Verification items for the finished model (mm, model axes). A direction names the side the tool comes from. Round coordinates to 2 decimals unless told otherwise and drop trailing zeros. Loops run counter-clockwise (first coordinate to the right, second up) from the corner with the lowest first, then second, coordinate; pieces in that order, holes last. Notation, with made-up numbers: (89.25, -36.5) -> (98.25, -36.5) arc R6 cw to (98.25, -25.5) -> close; hole circle Ø5 at (-11, 42). An arc over 180 degrees is marked (long way). Write item = value, one per line.
```python
from build123d import *

# Parameters (mm, degrees)
SKETCH1_R           = 78.35
SKETCH1_R_2         = 4
SKETCH1_R_3         = 3
BOSS_EXTRUDE1_DEPTH = 5
SKETCH2_R           = 78.35
SKETCH2_R_2         = 75.35
BOSS_EXTRUDE2_DEPTH = 8
SKETCH3_W           = 100
SKETCH3_H           = 100
CUT_EXTRUDE1_DEPTH  = 3


with BuildPart() as part:
    # Sketch1 → Boss-Extrude1 (new body)
    with BuildSketch(Plane(origin=(0, 0, 0), x_dir=(1, 0, 0), z_dir=(0, 1, 0))):
        with Locations(Location((0, 0, 0), (0, 0, 270))):
            Circle(SKETCH1_R)
        with Locations(Location((-62.5, 0, 0), (0, 0, 270))):
            Circle(SKETCH1_R_2, mode=Mode.SUBTRACT)
        with Locations(Location((62.5, 0, 0), (0, 0, 270))):
            Circle(SKETCH1_R_2, mode=Mode.SUBTRACT)
        with Locations(Location((0, 62.5, 0), (0, 0, 270))):
            Circle(SKETCH1_R_3, mode=Mode.SUBTRACT)
        with Locations(Location((0, -62.5, 0), (0, 0, 270))):
            Circle(SKETCH1_R_3, mode=Mode.SUBTRACT)
    extrude(amount=BOSS_EXTRUDE1_DEPTH)

    # Sketch2 → Boss-Extrude2 (add)
    with BuildSketch(Plane(origin=(0, 5, 0), x_dir=(1, 0, 0), z_dir=(0, 1, 0))):
        with Locations(Location((0, 0, 0), (0, 0, 270))):
            Circle(SKETCH2_R)
        with Locations(Location((0, 0, 0), (0, 0, 270))):
            Circle(SKETCH2_R_2, mode=Mode.SUBTRACT)
    extrude(amount=BOSS_EXTRUDE2_DEPTH)

    # Sketch3 → Cut-Extrude1 (cut)
    with BuildSketch(Plane(origin=(0, 5, 0), x_dir=(1, 0, 0), z_dir=(0, 1, 0))):
        Rectangle(SKETCH3_W, SKETCH3_H)
    extrude(amount=-CUT_EXTRUDE1_DEPTH, mode=Mode.SUBTRACT)


solid = part.part
```
(1) Draft check along X on faces 1 (the face through (64, 13, -41)), 2 (the face through (-1.8, 2.5, -64.9)), 3 (the face through (23.534, 6.409, 74.732)). Enter one of: released by +X, released by -X, zero draft, split by the parting line, or undercut.
Filled sheet:
face_1 = zero draft
face_2 = undercut
face_3 = split by the parting line
(2) Set-up check for faces 4 (the face through (74.71, 8.94, -9.81)), 5 (the face through (1, 0, -1)): record each of +Z, -Z, +X, -X, +Y, -Y from which the full face is reachable in a straight line by a thin tool's end or side.
Filled sheet:
face_4 = +Y
face_5 = +Z, -Z, +X, -X, -Y
(3) Material ranges on probe 1 along X at (y, z) = (1.25, 0); probe 2 along X at (y, z) = (3.2, 0); probe 3 along X at (y, z) = (9.5, 0), recorded low to high. Write a range as from..to.
Filled sheet:
probe_1 = -78.35..-66.5, -58.5..58.5, 66.5..78.35
probe_2 = -78.35..-66.5, -58.5..-50, 50..58.5, 66.5..78.35
probe_3 = -78.35..-75.35, 75.35..78.35
(4) Sectioned sample at A-A, the plane z = 0. Record the cut outline in (x, y).
Filled sheet:
outline = (-78.35, 0) -> (-66.5, 0) -> (-66.5, 5) -> (-75.35, 5) -> (-75.35, 13) -> (-78.35, 13) -> close; (-58.5, 0) -> (58.5, 0) -> (58.5, 5) -> (50, 5) -> (50, 2) -> (-50, 2) -> (-50, 5) -> (-58.5, 5) -> close; (66.5, 0) -> (78.35, 0) -> (78.35, 13) -> (75.35, 13) -> (75.35, 5) -> (66.5, 5) -> close
(5) Sectioned sample at C-C, the plane z = -62.5. Record the cut outline in (x, y).
Filled sheet:
outline = (-47.25, 0) -> (-3, 0) -> (-3, 5) -> (-42.09, 5) -> (-42.09, 13) -> (-47.25, 13) -> close; (3, 0) -> (47.25, 0) -> (47.25, 13) -> (42.09, 13) -> (42.09, 5) -> (3, 5) -> close
(6) Sectioned sample at B-B, the plane x = 0. Record the cut outline in (y, z), and give its area (4 significant figures).
Filled sheet:
outline = (0, -78.35) -> (13, -78.35) -> (13, -75.35) -> (5, -75.35) -> (5, -65.5) -> (0, -65.5) -> close; (0, -59.5) -> (5, -59.5) -> (5, -50) -> (2, -50) -> (2, 50) -> (5, 50) -> (5, 59.5) -> (0, 59.5) -> close; (0, 65.5) -> (5, 65.5) -> (5, 75.35) -> (13, 75.35) -> (13, 78.35) -> (0, 78.35) -> close
area = 471.5 mm2
(7) Go/stop test with flat-tipped pins: pin 1 Ø6 at (x, y) = (-10.5, 6.5) entering from +Z; pin 2 Ø3.5 at (x, y) = (11.5, 4) entering from +Z; pin 3 Ø4 at (x, z) = (1, 13.5) entering from +Y; pin 4 Ø6.5 at (x, z) = (-62.5, 0) entering from +Y. Record where each tip stops, or that it passes through.
Filled sheet:
pin_1 = 77.99
pin_2 = 77.74
pin_3 = 2
pin_4 = through
(8) Sectioned sample at D-D, the plane y = 8.5. Record the cut outline in (x, z).
Filled sheet:
outline = circle Ø156.7 at (0, 0); hole circle Ø150.7 at (0, 0)
